The listing builds one solid part. Answer for the finished solid, in the listing's coordinates (mm). A direction names the side the tool comes from. Give positions to 0.01 mm unless a question says otherwise; leave off trailing zeros. Order: outer loops, then holes, each group sorted by start corner. A loop starts at its lowest first (then second) coordinate and runs counter-clockwise, first axis right, second up. Notation, with made-up numbers: (9, 88.5) - (35, 88.5) arc R22 ccw to (35, 110.5) - close; hole circle Ø9 at (16, 47). An arc over 180 degrees is marked (long way). Write each question's results on one line, items separated by ' | '. Start each with the question number.
1. Section B-B (z = 6.25) is taken. Give the vertices of the cut face in (x, y), and give its area (3 significant figures).
2. Determine the mould class of faces 3 (the face through (-3.147, 31.217, 5.423)), 4 (the face through (10, 28, 5)), 5 (the face through (23.25, -0.34, 5.42)) for opening direction X: released by +X, released by -X, zero draft, split by the parting line, or undercut.
3. Section A-A (x = 9) is taken. Give the vertices of the cut face in (y, z).
4. Which of the six approach directions +Z, -Z, +X, -X, +Y, -Y give full straight-line access (tool end or side, diameter ignored) to faces 1 (the face through (10, 0, 5)), 2 (the face through (9, -4.5, 5))?
5. Section C-C (x = 20.25) is taken. Give the vertices of the cut face in (y, z).
6. Section D-D (y = -1) is taken. Give the vertices of the cut face in (x, z), and give its area (3 significant figures).
7. Flat-ended cylindrical pins translate along their axes: pin 1 (3 mm diameter, centred on y = 16, z = 7, fed in from +X); pin 2 (2 mm diameter, centred on y = 24, z = 10, fed in from +X). Find the tip coordinate at first contact, or state that the pin passes through.
8. Find the intervals of material crossed by L1, parallel to Y at x = 5.5, z = 4.75; L2, parallel to X at y = 17, z = 1; L3, parallel to X at y = 3.5, z = 6.5, in increasing order.
from build123d import *

# Parameters (mm, degrees)
F1_DEPTH = 11


with BuildPart() as f1:
    # F0 (on Top) → F1 (new body)
    with BuildSketch(Plane.XY):
        with BuildLine():
            Line((19, 0), (0, 0))
            Line((0, 0), (0, 28))
            Line((0, 28), (21, 28))
            Line((21, 28), (21, 24))
            ThreePointArc((21, 24), (25.25, 28.25), (21, 32.5))
            Line((21, 32.5), (0, 32.5))
            ThreePointArc((0, 32.5), (-3.181981, 31.181981), (-4.5, 28))
            Line((-4.5, 28), (-4.5, 0))
            ThreePointArc((-4.5, 0), (-3.181981, -3.181981), (0, -4.5))
            Line((0, -4.5), (19, -4.5))
            ThreePointArc((19, -4.5), (23.25, -0.25), (19, 4))
            Line((19, 4), (19, 0))
        make_face()
    extrude(amount=F1_DEPTH)


solid = f1.part
Reported:
1) outline: (-4.5, 0) arc R4.5 ccw to (0, -4.5) - (19, -4.5) arc R4.25 ccw to (19, 4) - (19, 0) - (0, 0) - (0, 28) - (21, 28) - (21, 24) arc R4.25 ccw to (21, 32.5) - (0, 32.5) arc R4.5 ccw to (-4.5, 28) - close | area: 395 mm²
2) face 3: released by -X | face 4: undercut | face 5: released by +X
3) outline: (-4.5, 0) - (0, 0) - (0, 11) - (-4.5, 11) - close; (28, 0) - (32.5, 0) - (32.5, 11) - (28, 11) - close
4) face 1: +Z, -Z | face 2: +Z, -Z, +X, -X, -Y
5) outline: (-4.31, 0) - (3.81, 0) - (3.81, 11) - (-4.31, 11) - close; (28, 0) - (32.5, 0) - (32.5, 11) - (28, 11) - close
6) outline: (-4.39, 0) - (23.18, 0) - (23.18, 11) - (-4.39, 11) - close | area: 303 mm²
7) pin 1: x = 0 | pin 2: x = 23.74
8) L1: -4.5 to 0, 28 to 32.5 | L2: -4.5 to 0 | L3: -4.5 to 0, 19 to 21
